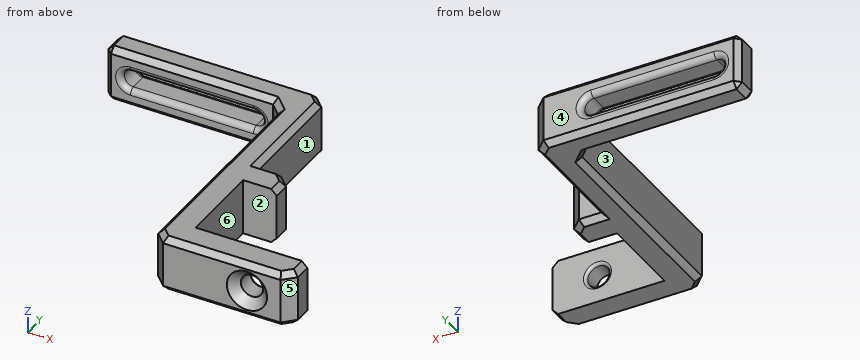
```python
from build123d import *

# Parameters (mm, degrees)
RESSALTO_EXTRUS_O1_DEPTH = 10
ESBO_O3_R                = 2
CORTE_EXTRUS_O1_DEPTH    = 15
CHANFRO1_SIZE            = 1.6
FILETE1_R                = 0.5
CHANFRO5_SIZE            = 2
CHANFRO8_SIZE            = 1
CORTE_EXTRUS_O3_DEPTH    = 10
FILETE3_R                = 1


with BuildPart() as part:
    # Esboço1 → Ressalto-extrusão1 (new body)
    with BuildSketch(Plane.XY):
        Polygon((1.886382163, -7.75), (-4.113617837, -7.75), (-4.113617837, -22.95), (15.886382163, -22.95), (15.886382163, -27.95), (-9.113617837, -27.95), (-9.113617837, 14.25), (-41.113617837, 14.25), (-41.113617837, 19.25), (-4.113617837, 19.25), (-4.113617837, -2.75), (1.886382163, -2.75), align=None)
    extrude(amount=RESSALTO_EXTRUS_O1_DEPTH)

    # Esboço3 → Corte-extrusão1 (cut)
    with BuildSketch(Plane.XZ.offset(27.95)):
        with Locations(Location((7.886382163, 5, 0), (0, 0, 270))):
            Circle(ESBO_O3_R)
    extrude(amount=-CORTE_EXTRUS_O1_DEPTH, mode=Mode.SUBTRACT)

    # Chanfro1
    chanfro1_edges = [part.edges().sort_by_distance(p)[0] for p in [
        (7.886382163, -27.95, 7),
    ]]
    chamfer(chanfro1_edges, length=CHANFRO1_SIZE)

    # Filete1
    filete1_edges = [part.edges().sort_by_distance(p)[0] for p in [
        (7.886382163, -22.95, 7),
    ]]
    fillet(filete1_edges, radius=FILETE1_R)

    # Chanfro5
    chanfro5_edges = [part.edges().sort_by_distance(p)[0] for p in [
        (15.886382163, -27.95, 5),
        (-9.113617837, -27.95, 5),
        (-9.113617837, 14.25, 5),
        (-4.113617837, 19.25, 5),
        (1.886382163, -2.75, 5),
    ]]
    chamfer(chanfro5_edges, length=CHANFRO5_SIZE)

    # Chanfro8
    chanfro8_edges = [part.edges().sort_by_distance(p)[0] for p in [
        (-4.113617837, 7.25, 10),
        (-26.113617837, 14.25, 0),
        (-41.113617837, 16.75, 0),
        (-4.113617837, 7.25, 0),
        (1.886382163, -6.25, 0),
        (-41.113617837, 16.75, 10),
        (-41.113617837, 14.25, 5),
        (-41.113617837, 19.25, 5),
        (-26.113617837, 14.25, 10),
        (-9.113617837, -6.85, 0),
        (1.886382163, -6.25, 10),
        (-9.113617837, -6.85, 10),
        (-23.613617837, 19.25, 0),
        (-23.613617837, 19.25, 10),
        (15.886382163, -24.45, 0),
        (3.386382163, -27.95, 0),
        (-2.113617837, -2.75, 0),
        (0.886382163, -3.75, 0),
        (14.886382163, -26.95, 0),
        (-8.113617837, -26.95, 0),
        (-5.113617837, 18.25, 0),
        (-2.113617837, -2.75, 10),
        (3.386382163, -27.95, 10),
        (15.886382163, -24.45, 10),
        (0.886382163, -3.75, 10),
        (14.886382163, -26.95, 10),
        (-8.113617837, -26.95, 10),
        (-5.113617837, 18.25, 10),
        (-10.113617837, 13.25, 0),
        (-10.113617837, 13.25, 10),
    ]]
    chamfer(chanfro8_edges, length=CHANFRO8_SIZE)

    # Esboço4 → Corte-extrusão3 (cut)
    with BuildSketch(Plane.XZ.offset(-14.25)):
        with BuildLine():
            Line((-36.613617837, 6.65), (-14.613617837, 6.65))
            ThreePointArc((-14.613617837, 6.65), (-12.963617837, 5), (-14.613617837, 3.35))
            Line((-14.613617837, 3.35), (-36.613617837, 3.35))
            ThreePointArc((-36.613617837, 3.35), (-38.263617837, 5), (-36.613617837, 6.65))
        make_face()
    extrude(amount=-CORTE_EXTRUS_O3_DEPTH, mode=Mode.SUBTRACT)

    # Filete3
    filete3_edges = [part.edges().sort_by_distance(p)[0] for p in [
        (-38.263617837, 19.25, 5),
        (-25.613617837, 19.25, 6.65),
        (-12.963617837, 19.25, 5),
        (-25.613617837, 19.25, 3.35),
        (-38.263617837, 14.25, 5),
        (-25.613617837, 14.25, 3.35),
        (-12.963617837, 14.25, 5),
        (-25.613617837, 14.25, 6.65),
    ]]
    fillet(filete3_edges, radius=FILETE3_R)


solid = part.part
```
Input: part model. Units: mm. Frame: model coordinates. Face numbers are marked on the shaded views. A direction names the side the tool comes from. Give positions to 0.01 mm unless a question says otherwise; leave off trailing zeros. Order: outer loops, then holes, each group sorted by start corner. A loop starts at its lowest first (then second) coordinate and runs counter-clockwise, first axis right, second up. Notation, with made-up numbers: M 35.5,35 L 78.5,35 A13 ccw 78.5,57 Z; hole C -33.75,76.25 d1. An arc over 180 degrees is marked long. Return JSON: item names as keys, results as strings.
1) Mould query, pull axis Y, two halves, no side actions, for the marked faces 4, 5 and 6. Classes: released by +Y, released by -Y, zero draft, split by the parting line, or undercut.
Taken from the geometry:
{"face 4": "released by +Y", "face 5": "released by -Y", "face 6": "undercut"}
2) Section query B-B on y = -6. Output: boundary loops of the cut face in (x, z), and give its area (3 significant figures).
Taken from the geometry:
{"outline": "M -9.11,1 L -8.11,0 L 0.89,0 L 1.89,1 L 1.89,9 L 0.89,10 L -8.11,10 L -9.11,9 Z", "area": "108 mm2"}
3) Line query: L1, parallel to X at y = -25.5, z = 5; L2, parallel to X at y = 10.5, z = 3.5; L3, parallel to Y at x = -12, z = 7.5. Output: solid intervals per line, ascending. Write a range as [from, to].
Taken from the geometry:
{"L1": "x = [-9.11, 5.89], [9.89, 15.89]", "L2": "x = [-9.11, -4.11]", "L3": "y = [14.25, 19.25]"}
4) Access query for the marked faces 1, 2 and 3. Directions: +Z, -Z, +X, -X, +Y, -Y. A direction counts if a zero-diameter tool reaches every point of the face in a straight line with its end or side. Return the directions, or none.
Taken from the geometry:
{"face 1": "+Z, -Z, +X, +Y", "face 2": "+Z, -Z, +X", "face 3": "+Z, -Z, -X, -Y"}
5) Contact query for flat-ended pins moving along their axis: pin 1 (3 mm diameter, centred on x = -34, z = 5.5, fed in from +Y); pin 2 (2.5 mm diameter, centred on x = -19.5, z = 7, fed in from -Y); pin 3 (3.5 mm diameter, centred on y = -6, z = 4, fed in from +X). Output: stop coordinate, or through.
Taken from the geometry:
{"pin 1": "stops at y = 19.01", "pin 2": "stops at y = 14.25", "pin 3": "stops at x = 1.89"}
6) Section query A-A on x = -26. Output: boundary loops of the cut face in (y, z).
Taken from the geometry:
{"outline": "M 14.25,1 L 15.25,0 L 18.25,0 L 19.25,1 L 19.25,2.35 A1 ccw 18.25,3.35 L 15.25,3.35 A1 ccw 14.25,2.35 Z; M 14.25,7.65 A1 ccw 15.25,6.65 L 18.25,6.65 A1 ccw 19.25,7.65 L 19.25,9 L 18.25,10 L 15.25,10 L 14.25,9 Z"}
7) Section query C-C on z = 5. Count the separate pieces of the cut face and the enclosed holes in it, and give its area (3 significant figures).
Taken from the geometry:
{"separate pieces": "3", "enclosed holes": "0", "area": "369 mm2"}
8) Section query D-D on y = -11.5. Output: boundary loops of the cut face in (x, z), and give its area (3 significant figures).
Taken from the geometry:
{"outline": "M -9.11,1 L -8.11,0 L -4.11,0 L -4.11,10 L -8.11,10 L -9.11,9 Z", "area": "49.0 mm2"}
